from build123d import *

# Parameters (mm, degrees)
BOSS_EXTRUDE1_DEPTH     = 80
SKETCH2_R               = 20
CUT_EXTRUDE1_DEPTH      = 80
SKETCH4_W               = 20
SKETCH4_H               = 60
CUT_EXTRUDE3_DEPTH      = 170
CUT_EXTRUDE3_DEPTH_BACK = 60
SKETCH5_W               = 20
SKETCH5_H               = 10
CUT_EXTRUDE4_DEPTH      = 170
CUT_EXTRUDE4_DEPTH_BACK = 170
SKETCH6_W               = 60
SKETCH6_H               = 25
CUT_EXTRUDE5_DEPTH      = 30
SKETCH7_W               = 26.45751311
SKETCH7_H               = 10
SKETCH7_W_2             = 16.771243445
CUT_EXTRUDE6_DEPTH      = 62
SKETCH8_W               = 60
SKETCH8_H               = 25
BOSS_EXTRUDE2_DEPTH     = 30
CUT_EXTRUDE7_DEPTH      = 30
CUT_EXTRUDE8_DEPTH      = 30
CUT_EXTRUDE9_DEPTH      = 10
BOSS_EXTRUDE3_DEPTH     = 10
BOSS_EXTRUDE4_DEPTH     = 20
SKETCH18_W              = 37.195082215
SKETCH18_H              = 5
CUT_EXTRUDE23_DEPTH     = 20
CUT_EXTRUDE25_DEPTH     = 30
SKETCH21_W              = 30
SKETCH21_H              = 25.000260328
CUT_EXTRUDE31_DEPTH     = 30
CUT_EXTRUDE32_DEPTH     = 30
SKETCH26_W              = 10
SKETCH26_H              = 5.000052065
CUT_EXTRUDE33_DEPTH     = 57
SKETCH29_W              = 34.732287975
SKETCH29_H              = 30
CUT_EXTRUDE37_DEPTH     = 57
SKETCH30_W              = 34.732287975
SKETCH30_H              = 10
CUT_EXTRUDE38_DEPTH     = 57
SKETCH31_W              = 10
SKETCH31_H              = 0.158503964
CUT_EXTRUDE39_DEPTH     = 57
SKETCH32_W              = 0.091268964
SKETCH32_H              = 10
CUT_EXTRUDE40_DEPTH     = 57
BOSS_EXTRUDE6_DEPTH     = 30
BOSS_EXTRUDE7_DEPTH     = 10
SKETCH37_W              = 20
SKETCH37_H              = 70
CUT_EXTRUDE47_DEPTH     = 68
SKETCH45_W              = 60
SKETCH45_H              = 30
BOSS_EXTRUDE10_DEPTH    = 0.0001
BOSS_EXTRUDE11_DEPTH    = 20
SKETCH49_W              = 20
SKETCH49_H              = 70
CUT_EXTRUDE54_DEPTH     = 95


with BuildPart() as part:
    # Sketch1 → Boss-Extrude1 (new body)
    with BuildSketch(Plane.XY):
        with BuildLine():
            Line((0, 40), (60, 40))
            ThreePointArc((60, 40), (100, 0), (60, -40))
            Line((60, -40), (0, -40))
            ThreePointArc((0, -40), (-40, 0), (0, 40))
        make_face()
    extrude(amount=BOSS_EXTRUDE1_DEPTH)

    # Sketch2 → Cut-Extrude1 (cut)
    with BuildSketch(Plane.XY.offset(80)):
        with Locations((30, 0)):
            Circle(SKETCH2_R)
    extrude(amount=-CUT_EXTRUDE1_DEPTH, mode=Mode.SUBTRACT)

    # Sketch4 → Cut-Extrude3 (cut, two sides)
    with BuildSketch(Plane(origin=(0, 0, 0), x_dir=(0, 0, -1), z_dir=(1, 0, 0))) as cut_extrude3_sk:
        with Locations((-70, 10)):
            Rectangle(SKETCH4_W, SKETCH4_H)
    extrude(amount=CUT_EXTRUDE3_DEPTH, mode=Mode.SUBTRACT)
    extrude(cut_extrude3_sk.sketch, amount=-CUT_EXTRUDE3_DEPTH_BACK, mode=Mode.SUBTRACT)

    # Sketch5 → Cut-Extrude4 (cut, two sides)
    with BuildSketch(Plane(origin=(0, 0, 0), x_dir=(0, 0, -1), z_dir=(1, 0, 0))) as cut_extrude4_sk:
        with Locations((-50, 35)):
            Rectangle(SKETCH5_W, SKETCH5_H)
    extrude(amount=CUT_EXTRUDE4_DEPTH, mode=Mode.SUBTRACT)
    extrude(cut_extrude4_sk.sketch, amount=-CUT_EXTRUDE4_DEPTH_BACK, mode=Mode.SUBTRACT)

    # Sketch6 → Cut-Extrude5 (cut)
    with BuildSketch(Plane.XY.offset(80)):
        with Locations((30, -27.5)):
            Rectangle(SKETCH6_W, SKETCH6_H)
    extrude(amount=-CUT_EXTRUDE5_DEPTH, mode=Mode.SUBTRACT)

    # Sketch7 → Cut-Extrude6 (cut)
    with BuildSketch(Plane.XZ.offset(15)):
        with Locations((30, 55)):
            Rectangle(SKETCH7_W, SKETCH7_H)
        with Locations((51.614378278, 55)):
            Rectangle(SKETCH7_W_2, SKETCH7_H)
        with Locations((8.385621722, 55)):
            Rectangle(SKETCH7_W_2, SKETCH7_H)
    extrude(amount=-CUT_EXTRUDE6_DEPTH, mode=Mode.SUBTRACT)

    # Sketch8 → Boss-Extrude2 (add)
    with BuildSketch(Plane.XY.offset(50)):
        with Locations((30, -27.5)):
            Rectangle(SKETCH8_W, SKETCH8_H)
    extrude(amount=BOSS_EXTRUDE2_DEPTH)

    # Sketch9 → Cut-Extrude7 (cut)
    with BuildSketch(Plane(origin=(0, 0, 50), x_dir=(-1, 0, 0), z_dir=(0, 0, -1))):
        with BuildLine():
            Line((-43.228756555, -15), (-16.771243445, -15))
            ThreePointArc((-16.771243445, -15), (-30, -20), (-43.228756555, -15))
        make_face()
    extrude(amount=-CUT_EXTRUDE7_DEPTH, mode=Mode.SUBTRACT)

    # Sketch10 → Cut-Extrude8 (cut)
    with BuildSketch(Plane.XY.offset(80)):
        with BuildLine():
            Line((60, -20), (60, -40))
            ThreePointArc((60, -40), (80, -34.641016151), (94.641016151, -20))
            Line((94.641016151, -20), (60, -20))
        make_face()
    extrude(amount=-CUT_EXTRUDE8_DEPTH, mode=Mode.SUBTRACT)

    # Sketch11 → Cut-Extrude9 (cut)
    with BuildSketch(Plane.XY.offset(50)):
        with BuildLine():
            Line((60, 30), (0, 30))
            Line((0, 30), (0, -15))
            Line((0, -15), (16.771243445, -15))
            ThreePointArc((16.771243445, -15), (30, 20), (43.228756555, -15))
            Line((43.228756555, -15), (60, -15))
            Line((60, -15), (60, 30))
        make_face()
    extrude(amount=-CUT_EXTRUDE9_DEPTH, mode=Mode.SUBTRACT)

    # Sketch12 → Boss-Extrude3 (add)
    with BuildSketch(Plane.XY.offset(50)):
        with BuildLine():
            Line((60, -20), (94.641016151, -20))
            ThreePointArc((94.641016151, -20), (80, -34.641016151), (60, -40))
            Line((60, -40), (60, -20))
        make_face()
    extrude(amount=BOSS_EXTRUDE3_DEPTH)

    # Sketch17 → Boss-Extrude4 (add)
    with BuildSketch(Plane.XY.offset(60)):
        with BuildLine():
            Line((97.080992435, -15), (60, -15))
            Line((60, -15), (60, -40))
            ThreePointArc((60, -40), (82.360679775, -33.166247904), (97.080992435, -15))
        make_face()
    extrude(amount=BOSS_EXTRUDE4_DEPTH)

    # Sketch18 → Cut-Extrude23 (cut)
    with BuildSketch(Plane.XY.offset(80)):
        with Locations((78.483451328, -17.5)):
            Rectangle(SKETCH18_W, SKETCH18_H)
    extrude(amount=-CUT_EXTRUDE23_DEPTH, mode=Mode.SUBTRACT)

    # Sketch19 → Cut-Extrude25 (cut)
    with BuildSketch(Plane.XY.offset(80)):
        with BuildLine():
            Line((16.771243445, -15), (0, -15))
            Line((0, -15), (0, -20))
            Line((0, -20), (0, -40))
            Line((0, -40), (60, -40))
            Line((60, -40), (59.908728176, -20))
            Line((59.908728176, -20), (59.88591022, -20))
            Line((59.88591022, -20), (59.88591022, -15))
            Line((59.88591022, -15), (43.228756555, -15))
            ThreePointArc((43.228756555, -15), (30, -20), (16.771243445, -15))
        make_face()
    extrude(amount=-CUT_EXTRUDE25_DEPTH, mode=Mode.SUBTRACT)

    # Sketch21 → Cut-Extrude31 (cut)
    with BuildSketch(Plane(origin=(59.816210597, 0.272976733, 0), x_dir=(0, 0, 1), z_dir=(-0.999989587, -0.004563544, 0))):
        with Locations((65, -27.773265937)):
            Rectangle(SKETCH21_W, SKETCH21_H)
    extrude(amount=CUT_EXTRUDE31_DEPTH, mode=Mode.SUBTRACT)

    # Sketch24 → Cut-Extrude32 (cut)
    with BuildSketch(Plane.XY.offset(50)):
        with BuildLine():
            Line((59.88591022, -15), (97.080992435, -15))
            ThreePointArc((97.080992435, -15), (98.92976522, 9.1909401), (86.456775103, 30.000650845))
            Line((86.456775103, 30.000650845), (59.88591022, 30.000650845))
            Line((59.88591022, 30.000650845), (59.88591022, -15))
        make_face()
    extrude(amount=CUT_EXTRUDE32_DEPTH, mode=Mode.SUBTRACT)

    # Sketch26 → Cut-Extrude33 (cut)
    with BuildSketch(Plane(origin=(59.816210597, 0.272976733, 0), x_dir=(0, 0, 1), z_dir=(-0.999989587, -0.004563544, 0))):
        with Locations((55, -17.773161806)):
            Rectangle(SKETCH26_W, SKETCH26_H)
    extrude(amount=-CUT_EXTRUDE33_DEPTH, mode=Mode.SUBTRACT)

    # Sketch29 → Cut-Extrude37 (cut)
    with BuildSketch(Plane(origin=(0, -20, 0), x_dir=(1, 0, 0), z_dir=(0, 1, 0))):
        with Locations((77.274872164, -65)):
            Rectangle(SKETCH29_W, SKETCH29_H)
    extrude(amount=-CUT_EXTRUDE37_DEPTH, mode=Mode.SUBTRACT)

    # Sketch30 → Cut-Extrude38 (cut)
    with BuildSketch(Plane.XZ.offset(20)):
        with Locations((77.274872164, 55)):
            Rectangle(SKETCH30_W, SKETCH30_H)
    extrude(amount=-CUT_EXTRUDE38_DEPTH, mode=Mode.SUBTRACT)

    # Sketch31 → Cut-Extrude39 (cut)
    with BuildSketch(Plane.ZY.offset(-94.641016151)):
        with Locations((55, -19.920748018)):
            Rectangle(SKETCH31_W, SKETCH31_H)
    extrude(amount=-CUT_EXTRUDE39_DEPTH, mode=Mode.SUBTRACT)

    # Sketch32 → Cut-Extrude40 (cut)
    with BuildSketch(Plane(origin=(0.092517579, -20.272976733, 0), x_dir=(0.999989587, 0.004563544, 0), z_dir=(-0.004563544, 0.999989587, 0))):
        with Locations((94.5951176, -55)):
            Rectangle(SKETCH32_W, SKETCH32_H)
    extrude(amount=-CUT_EXTRUDE40_DEPTH, mode=Mode.SUBTRACT)

    # Sketch33 → Boss-Extrude6 (add)
    with BuildSketch(Plane.XY.offset(50)):
        with BuildLine():
            Line((60, -20), (60, -40))
            ThreePointArc((60, -40), (80, -34.641016151), (94.641016151, -20))
            Line((94.641016151, -20), (60, -20))
        make_face()
    extrude(amount=BOSS_EXTRUDE6_DEPTH)

    # Sketch34 → Boss-Extrude7 (add)
    with BuildSketch(Plane.XY.offset(50)):
        with BuildLine():
            Line((60, 30), (60, -20))
            Line((60, -20), (94.641016151, -20))
            ThreePointArc((94.641016151, -20), (99.474771304, 6.46083822), (86.457513111, 30))
            Line((86.457513111, 30), (60, 30))
        make_face()
    extrude(amount=BOSS_EXTRUDE7_DEPTH)

    # Sketch37 → Cut-Extrude47 (cut)
    with BuildSketch(Plane(origin=(0, 0, 0), x_dir=(0, 0, -1), z_dir=(1, 0, 0))):
        with Locations((-10, -5)):
            Rectangle(SKETCH37_W, SKETCH37_H)
    extrude(amount=-CUT_EXTRUDE47_DEPTH, mode=Mode.SUBTRACT)

    # Sketch45 → Boss-Extrude10 (add)
    with BuildSketch(Plane(origin=(0, -40, 0), x_dir=(-1, 0, 0), z_dir=(0, -1, 0))):
        with Locations((-30, -65)):
            Rectangle(SKETCH45_W, SKETCH45_H)
    extrude(amount=-BOSS_EXTRUDE10_DEPTH)

    # Sketch46 → Boss-Extrude11 (add)
    with BuildSketch(Plane(origin=(0, 0, 20), x_dir=(-1, 0, 0), z_dir=(0, 0, -1))):
        with BuildLine():
            Line((26.457513111, 30), (0, 30))
            Line((0, 30), (0, -40))
            ThreePointArc((0, -40), (37.416573868, -14.142135624), (26.457513111, 30))
        make_face()
    extrude(amount=BOSS_EXTRUDE11_DEPTH)

    # Sketch49 → Cut-Extrude54 (cut)
    with BuildSketch(Plane(origin=(0, 0, 0), x_dir=(0, 0, -1), z_dir=(1, 0, 0))):
        with Locations((-10, -5)):
            Rectangle(SKETCH49_W, SKETCH49_H)
    extrude(amount=-CUT_EXTRUDE54_DEPTH, mode=Mode.SUBTRACT)


solid = part.part
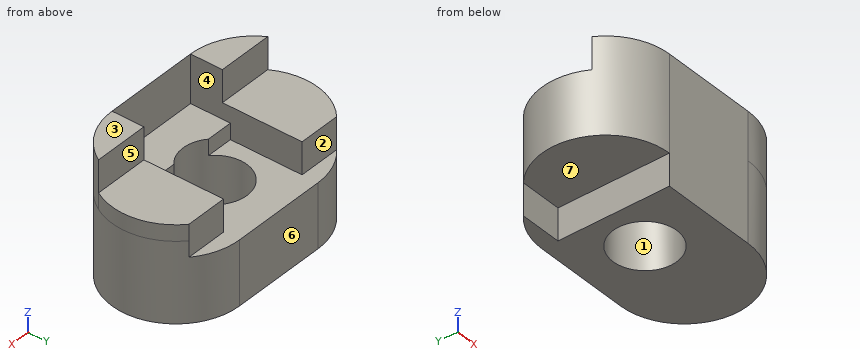
Work out the finished part from the listing and answer in its coordinate system (mm). Face numbers are marked on the shaded views. A direction names the side the tool comes from. Give positions to 0.01 mm unless a question says otherwise; leave off trailing zeros. Loops run counter-clockwise (first coordinate to the right, second up) from the corner with the lowest first, then second, coordinate; pieces in that order, holes last. Notation, with made-up numbers: (54, 24) -> (108, 24) arc R17 ccw to (108, 33) -> close; hole circle Ø7 at (-16, -2.75). An arc over 180 degrees is marked (long way). Use a Markdown table: item, result. Add a question column.
1) Each of these flat-tipped pins is pushed along its axis until it touches: P1, Ø22, axis at x = 69, z = 47.5, coming from the +Y side; P2, Ø20, axis at x = 39, y = -26.5, coming from the +Z side; P3, Ø3, axis at x = 6, z = 43.5, coming from the +Y side; P4, Ø1, axis at x = 27, y = -22, coming from the -Z side. Where does it stop, or does it pass through?
2) The part is cut by section C-C, the plane z = 18.5. Determine the outline of the cut face in (x, y), plus the area to 3 significant figures.
3) The part is cut by section D-D, the plane z = 64.5. Determine the outline of the cut face in (x, y).
4) For a pull along Y with two mould halves and no side action, classify the marked faces 1, 2 and 3 as +Y half, -Y half, draft (parallel to the pull), parting line (faces both ways), or undercut.
5) The part is cut by section A-A, the plane y = 0. Determine the outline of the cut face in (x, z), plus the area to 3 significant figures.
6) Which of the six approach directions +Z, -Z, +X, -X, +Y, -Y give full straight-line access (tool end or side, diameter ignored) to the marked faces 4, 5, 6 and 7?
7) Consider line 1 along Y through (x, z) = (30, 12); line 2 along X through (y, z) = (0, 17); line 3 along Z through (x, y) = (54, -2). Determine where each line is inside the solid, lowest interval first.
Reported:
| question | item | result |
|---|---|---|
| 1 | P1 | stops at y = 39.99 |
| 1 | P2 | stops at z = 50 |
| 1 | P3 | stops at y = -15 |
| 1 | P4 | stops at z = 0 |
| 2 | outline | (-26.46, 30) -> (0, 30) -> (0, -40) -> (60, -40) arc R40 ccw to (60, 40) -> (0, 40) arc R40 ccw to start; hole circle Ø40 at (30, 0) |
| 2 | area | 6,240 mm^2 |
| 3 | outline | (-34.64, -20) arc R40 ccw to (0, -40) -> (60, -40) arc R40 ccw to (94.64, -20) -> (60, -20) -> (60, -40) -> (0, -40) -> (0, -20) -> close |
| 4 | face 1 | undercut |
| 4 | face 2 | +Y half |
| 4 | face 3 | draft |
| 5 | outline | (-40, 20) -> (0, 20) -> (0, 0) -> (10, 0) -> (10, 40) -> (0, 40) -> (0, 60) -> (-40, 60) -> close; (50, 0) -> (100, 0) -> (100, 60) -> (60, 60) -> (60, 40) -> (50, 40) -> close |
| 5 | area | 4,800 mm^2 |
| 6 | face 4 | +Z, +Y |
| 6 | face 5 | +Z, +X, -X, +Y |
| 6 | face 6 | +Z, -Z, +X, -X, +Y |
| 6 | face 7 | -Z, -X, -Y |
| 7 | line 1 | y = -40 to -20, 20 to 40 |
| 7 | line 2 | x = 0 to 10, 50 to 100 |
| 7 | line 3 | z = 0 to 40 |
